```python
from build123d import *

# Parameters (mm, degrees)
SKETCH3_R           = 4.85
SKETCH3_R_2         = 4.15
BOSS_EXTRUDE1_DEPTH = 14.5
SKETCH4_R           = 2
CUT_EXTRUDE1_DEPTH  = 11.5
SKETCH5_R           = 2
CUT_EXTRUDE2_DEPTH  = 11.5


with BuildPart() as part:
    # Sketch3 → Boss-Extrude1 (new body)
    with BuildSketch(Plane.XY.offset(2)):
        Circle(SKETCH3_R)
        Circle(SKETCH3_R_2, mode=Mode.SUBTRACT)
    extrude(amount=BOSS_EXTRUDE1_DEPTH)

    # Sketch4 → Cut-Extrude1 (cut)
    with BuildSketch(Plane(origin=(-13.41400196, 54.908076208, -66.470187191), x_dir=(0, 1, 0), z_dir=(1, 0, 0))):
        with Locations((-54.908076208, 60.970187191)):
            Circle(SKETCH4_R)
        with Locations(Location((-54.908076208, 79.970187191, 0), (0, 0, 90))):
            Circle(SKETCH4_R)
    extrude(amount=CUT_EXTRUDE1_DEPTH, mode=Mode.SUBTRACT)

    # Sketch5 → Cut-Extrude2 (cut)
    with BuildSketch(Plane(origin=(0, -2, -8.5), x_dir=(1, 0, 0), z_dir=(0, 1, 0))):
        with Locations(Location((0, -22, 0), (0, 0, 270))):
            Circle(SKETCH5_R)
    extrude(amount=-CUT_EXTRUDE2_DEPTH, mode=Mode.SUBTRACT)


solid = part.part
```
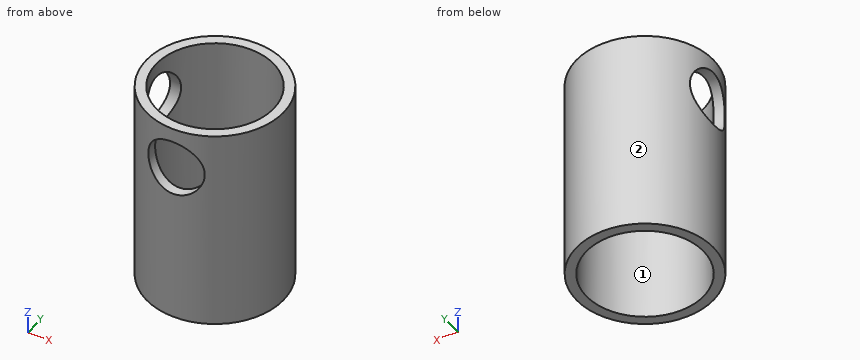
Source: CAD feature listing. Evaluate the final solid. Frame: model axes, mm. Face numbers are marked on the shaded views. Round coordinates to 2 decimals unless told otherwise and drop trailing zeros. Loops run counter-clockwise (first coordinate to the right, second up) from the corner with the lowest first, then second, coordinate; pieces in that order, holes last. Notation, with made-up numbers: M 84.25,24.25 L 106.25,24.25 A26 cw 106.25,39.25 Z; hole C 48,55.5 d2. An arc over 180 degrees is marked long. Put each result on its own line as item: value.
(1) Pull-direction query (Y, two-part tool) for the marked faces 1 and 2; classes: released by +Y, released by -Y, zero draft, split by the parting line, or undercut.
Solutions:
face 1: undercut
face 2: split by the parting line
(2) Section C-C, the plane z = 13.5. Return loops of the section in (x, y), and give its area (3 significant figures).
Solutions:
outline: M -4.42,-2 A4.85 ccw -2,-4.42 L -2,-3.64 A4.15 cw -3.64,-2 Z; M -4.42,2 L -3.64,2 A4.15 cw long 2,-3.64 L 2,-4.42 A4.85 ccw long Z
area: 14.0 mm²
(3) Section D-D, the plane x = -3.25. Return loops of the section in (y, z).
Solutions:
outline: M -3.6,2 L -2.58,2 L -2.58,16.5 L -3.6,16.5 Z; M 2.58,2 L 3.6,2 L 3.6,16.5 L 2.58,16.5 Z
(4) Section A-A, the plane y = 0. Return loops of the section in (x, z).
Solutions:
outline: M -4.85,2 L -4.15,2 L -4.15,11.5 L -4.85,11.5 Z; M -4.85,15.5 L -4.15,15.5 L -4.15,16.5 L -4.85,16.5 Z; M 4.15,2 L 4.85,2 L 4.85,16.5 L 4.15,16.5 Z
(5) First-contact query: pin 1 (3 mm diameter, centred on x = 0, z = 13.5, fed in from -Y); pin 2 (1.5 mm diameter, centred on y = -1.5, z = 4.5, fed in from +X); pin 3 (5 mm diameter, centred on y = 3.5, z = 4.5, fed in from +X). Flat tips, straight axial feed; report the tip coordinate or a pass-through.
Solutions:
pin 1: y = 3.87
pin 2: x = 4.79
pin 3: x = 4.75
(6) Ray query, line 1 (X direction, y = 0, z = 10.75); line 2 (X direction, y = 3.25, z = 3); line 3 (Y direction, x = 1.75, z = 7). Return the intervals inside material, ascending. Write a range as [from, to].
Solutions:
line 1: [-4.85, -4.15], [4.15, 4.85]
line 2: [-3.6, -2.58], [2.58, 3.6]
line 3: [-4.52, -3.76], [3.76, 4.52]
